The drawing under review shows one solid part. Ordinate dimensions are in mm from its lowest x, y, z. Give positions to 0.01 mm unless a question says otherwise; leave off trailing zeros. Write each loop counter-clockwise with the first axis right and the second up, starting at its lowest first coordinate (ties: lowest second). Pieces come first, ordered by that corner, then holes. Notation, with made-up numbers: (74.25, -16) -> (80.25, -16) arc R8 cw to (80.25, -8) -> close; hole circle Ø9 at (34.25, 13). An arc over 180 degrees is marked (long way). Use CSV: the item, a comma, the result in double quotes.
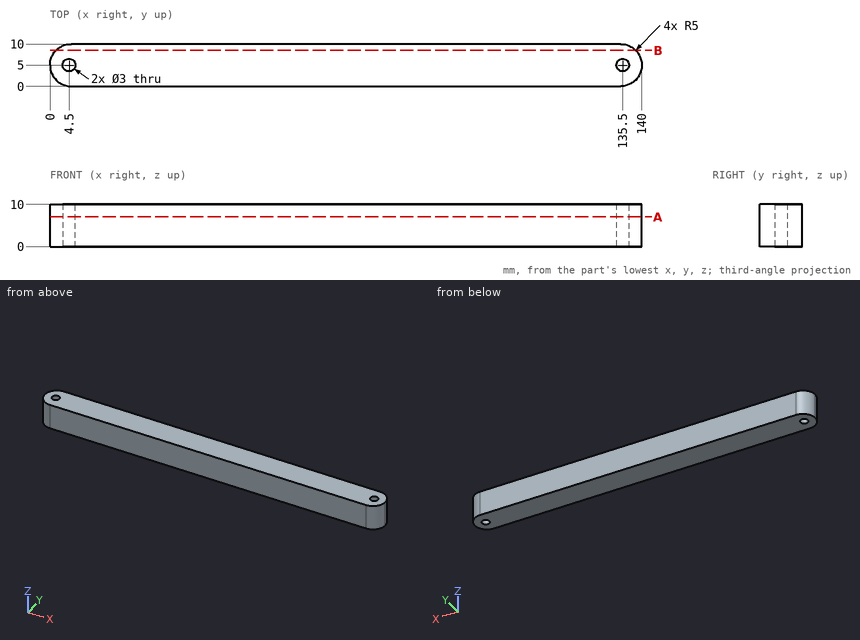
(1) Take a section at A-A (z = 7). State how many separate pieces and enclosed holes the cut face has, then the cut area to 3 significant figures.
Established:
separate pieces,"1"
enclosed holes,"2"
area,"1,360 mm2"
(2) For line 1 along X through (y, z) = (4, 5.25); line 2 along Y through (x, z) = (4.5, 4.25) (3 decimals); line 3 along X through (y, z) = (4.5, 3.75) (1 decimal), list the stretches that pass through material, from the lowest coordinate up. Write a range as [from, to].
Established:
line 1,"x = [0.1, 3.38], [5.62, 134.38], [136.62, 139.9]"
line 2,"y = [0.025, 3.5], [6.5, 9.975]"
line 3,"x = [0, 3.1], [5.9, 134.1], [136.9, 140]"
(3) Clearance check with a flat-ended pin moving along its axis: pin 1 (2.5 mm diameter, centred on x = 4.5, y = 5, fed in from -Z). State where the tip first meets the part, or that it passes through.
Established:
pin 1,"passes through"
(4) Take a section at B-B (y = 8.5). Write out the cut boundary in (x, z), then the cut area to 3 significant figures.
Established:
outline,"(1.43, 0) -> (138.57, 0) -> (138.57, 10) -> (1.43, 10) -> close"
area,"1,370 mm2"
